from build123d import *

# Parameters (mm, degrees)
SKETCH1_W                = 2
SKETCH1_H                = 9
BOSS_EXTRUDE2_DEPTH      = 7
BOSS_EXTRUDE4_DEPTH      = 3.5
BOSS_EXTRUDE4_DEPTH_BACK = 3.5
SKETCH2_R                = 2.5
BOSS_EXTRUDE3_DEPTH      = 2
CUT_EXTRUDE3_DEPTH       = 18.291616466
FILLET1_R                = 1
FILLET2_R                = 2
FILLET2_OF_MIRROR2_R     = 2
FILLET3_R                = 1


with BuildPart() as part:
    # Sketch1 → Boss-Extrude2 (new body)
    with BuildSketch(Plane.XY):
        Rectangle(SKETCH1_W, SKETCH1_H)
    boss_extrude2 = extrude(amount=BOSS_EXTRUDE2_DEPTH)

    # Sketch5 → Boss-Extrude4 (add, two sides: drawn at the far end of the back side and taken through both)
    with BuildSketch(Plane.XY.offset(3.5).offset(-BOSS_EXTRUDE4_DEPTH_BACK)):
        Polygon((-3.035, -1.4675), (-1, -1.4675), (-1, 1.4675), (-3.035, 1.4675), (-3.035, 1.9675), (-4.97, 1.9675), (-4.97, -1.9675), (-3.035, -1.9675), align=None)
    extrude(amount=BOSS_EXTRUDE4_DEPTH + BOSS_EXTRUDE4_DEPTH_BACK)

    # Sketch2 → Boss-Extrude3 (add)
    with BuildSketch(Plane.XY):
        with BuildLine():
            Line((-1, 4.5), (8.5, 4.5))
            ThreePointArc((8.5, 4.5), (13, 0), (8.5, -4.5))
            Line((8.5, -4.5), (-1, -4.5))
            Line((-1, -4.5), (-1, 4.5))
        make_face()
        with Locations((8.5, 0)):
            Circle(SKETCH2_R, mode=Mode.SUBTRACT)
    boss_extrude3 = extrude(amount=-BOSS_EXTRUDE3_DEPTH)

    # Sketch4 → Cut-Extrude3 (cut, through all)
    with BuildSketch(Plane(origin=(0, 4.5, 0), x_dir=(1, 0, 0), z_dir=(0, 1, 0))):
        Polygon((-1, 0), (1, 2), (-1, 2), align=None)
    cut_extrude3 = extrude(amount=-CUT_EXTRUDE3_DEPTH, mode=Mode.SUBTRACT)

    # Fillet1
    fillet1_edges = [part.edges().sort_by_distance(p)[0] for p in [
        (1, 0, 0),
    ]]
    fillet(fillet1_edges, radius=FILLET1_R)

    # Fillet2
    fillet2_edges = [part.edges().sort_by_distance(p)[0] for p in [
        (1, 0, -2),
    ]]
    fillet(fillet2_edges, radius=FILLET2_R)

    # Mirror2: Boss-Extrude2, Boss-Extrude3, Cut-Extrude3 across plane
    add(boss_extrude2.mirror(Plane.XY.offset(3.5)))
    add(boss_extrude3.mirror(Plane.XY.offset(3.5)))
    add(cut_extrude3.mirror(Plane.XY.offset(3.5)), mode=Mode.SUBTRACT)

    # Fillet2 of Mirror2
    fillet2_of_mirror2_edges = [part.edges().sort_by_distance(p)[0] for p in [
        (1, 0, 9),
    ]]
    fillet(fillet2_of_mirror2_edges, radius=FILLET2_OF_MIRROR2_R)

    # Fillet3
    fillet3_edges = [part.edges().sort_by_distance(p)[0] for p in [
        (1, 0, 7),
    ]]
    fillet(fillet3_edges, radius=FILLET3_R)


solid = part.part
Part model, mm, in its own coordinate system. A direction names the side the tool comes from. Give positions to 0.01 mm unless a question says otherwise; leave off trailing zeros. Write each loop counter-clockwise with the first axis right and the second up, starting at its lowest first coordinate (ties: lowest second). Pieces come first, ordered by that corner, then holes.
1) Cut at D-D on z = 4.5. Write the cut outline in (x, y) (1 decimal).
Resolved:
outline: (-5, -2) - (-3, -2) - (-3, -1.5) - (-1, -1.5) - (-1, -4.5) - (1, -4.5) - (1, 4.5) - (-1, 4.5) - (-1, 1.5) - (-3, 1.5) - (-3, 2) - (-5, 2) - close
2) Pin check, flat tips, straight feed: pin 1 (1.2 mm diameter, centred on x = -2, y = -0.5, fed in from +Z); pin 2 (2.5 mm diameter, centred on y = -2.5, z = 4, fed in from -X); pin 3 (2.5 mm diameter, centred on y = 0, z = 3.5, fed in from +X); pin 4 (2 mm diameter, centred on x = -3.5, z = 5, fed in from +Y). Stop position of each tip, or through.
Resolved:
pin 1: stops at z = 7
pin 2: stops at x = -4.97
pin 3: stops at x = 1
pin 4: stops at y = 1.97
3) Probe L1, parallel to X at y = 1.5, z = 3.5 (3 decimals); L2, parallel to Z at x = 2.75, y = 0.75; L3, parallel to Y at x = 8.5, z = 7.75. List the from-to ranges inside material, lowest first.
Resolved:
L1: x = -4.97 to -3.035, -1 to 1
L2: z = -2 to 0, 7 to 9
L3: y = -4.5 to -2.5, 2.5 to 4.5
4) Two-plate mould, pull along Z, no slides. Class faces 1 (the face through (0, 0, -1)), 2 (the face through (5, 0, 7)), 3 (the face through (1.285, 0.063, 0.301)), 4 (the face through (1.053, -0.063, 8.844)): released by +Z, released by -Z, zero draft, split by the parting line, or undercut.
Resolved:
face 1: released by -Z
face 2: undercut
face 3: undercut
face 4: released by +Z
5) Cut at A-A on y = 0. Write the cut outline in (x, z), then the cut area to 3 significant figures.
Resolved:
outline: (-4.97, 0) - (-1, 0) - (0.41, -1.41) arc R2 ccw to (1.83, -2) - (6, -2) - (6, 0) - (2, 0) arc R1 cw to (1, 1) - (1, 6) arc R1 cw to (2, 7) - (6, 7) - (6, 9) - (1.83, 9) arc R2 ccw to (0.41, 8.41) - (-1, 7) - (-4.97, 7) - close; (11, -2) - (13, -2) - (13, 0) - (11, 0) - close; (11, 7) - (13, 7) - (13, 9) - (11, 9) - close
area: 74.0 mm2
6) Cut at C-C on x = 6.5. Write the cut outline in (y, z).
Resolved:
outline: (-4.5, -2) - (-1.5, -2) - (-1.5, 0) - (-4.5, 0) - close; (-4.5, 7) - (-1.5, 7) - (-1.5, 9) - (-4.5, 9) - close; (1.5, -2) - (4.5, -2) - (4.5, 0) - (1.5, 0) - close; (1.5, 7) - (4.5, 7) - (4.5, 9) - (1.5, 9) - close
7) Cut at B-B on x = 3. Write the cut outline in (y, z), then the cut area to 3 significant figures.
Resolved:
outline: (-4.5, -2) - (4.5, -2) - (4.5, 0) - (-4.5, 0) - close; (-4.5, 7) - (4.5, 7) - (4.5, 9) - (-4.5, 9) - close
area: 36.0 mm2
8) Which spindle directions (+Z, -Z, +X, -X, +Y, -Y) get a long thin tool onto all of the face, cutting with end or side? Do faces 5 (the face through (-1, 3, 3)), 6 (the face through (-3, 0, 0)), 7 (the face through (-3, 0, 7)), 8 (the face through (1, 0, 3)), 9 (the face through (-2, -1.468, 3)). Say none if no direction does.
Resolved:
face 5: +Z, -Z, +Y
face 6: -Z, -X, +Y, -Y
face 7: +Z, -X, +Y, -Y
face 8: +X, +Y, -Y
face 9: +Z, -Z, -Y
